Work out the finished part from the listing and answer in its coordinate system (mm). Coordinates: 2 decimals unless noted, no trailing zeros. Loops run counter-clockwise (first coordinate to the right, second up) from the corner with the lowest first, then second, coordinate; pieces in that order, holes last. Notation, with made-up numbers: (27, 45.5) - (78, 45.5) arc R21 ccw to (78, 79.5) - close; hole circle Ø10 at (70, -27). An arc over 180 degrees is marked (long way). Write each question's results on one line, items separated by ' | '. Start each with the question number.
1. A cutting plane is placed at B-B on x = -85. Determine the outline of the cut face in (y, z), then the cut area to 3 significant figures.
2. Each of these flat-tipped pins is pushed along its axis until it touches: P1, Ø10, axis at x = -74.5, y = 95, coming from the -Z side; P2, Ø1.6, axis at x = -62.7, y = 109.08, coming from the -Z side; P3, Ø2.5, axis at x = -121.2, y = 144.58, coming from the -Z side. Where does it stop, or does it pass through?
3. Find the intervals of material crossed by line 1 along Y through (x, z) = (-60, 0.3); line 2 along X through (y, z) = (54, 1); line 3 along Y through (x, z) = (-23.5, 0.6), in increasing order. Write a range as [from, to].
4. A cutting plane is placed at C-C on y = 39.5. Determine the outline of the cut face in (x, z).
5. A cutting plane is placed at A-A on z = 0.55. Determine the outline of the cut face in (x, y), then the cut area to 3 significant figures.
from build123d import *

# Parameters (mm, degrees)
SKETCH1_R           = 1
BOSS_EXTRUDE1_DEPTH = 1.5
CHAMFER1_SIZE       = 1


with BuildPart() as part:
    # Sketch1 → Boss-Extrude1 (new body)
    with BuildSketch(Plane.XY):
        with BuildLine():
            Line((20.7161288, 151.924941972), (-143.43387189, 151.924941972))
            ThreePointArc((-143.43387189, 151.924941972), (-144.494532062, 151.485602143), (-144.93387189, 150.424941972))
            Line((-144.93387189, 150.424941972), (-144.93387189, 48.261817052))
            ThreePointArc((-144.93387189, 48.261817052), (-144.494532062, 47.20115688), (-143.43387189, 46.761817052))
            Line((-143.43387189, 46.761817052), (-38.493629317, 46.761817052))
            ThreePointArc((-38.493629317, 46.761817052), (-37.328943614, 46.60848327), (-36.243629317, 46.158931369))
            Line((-36.243629317, 46.158931369), (-4.017847382, 27.553367493))
            ThreePointArc((-4.017847382, 27.553367493), (-2.879618836, 27.403516854), (-1.968809299, 28.10240556))
            Line((-1.968809299, 28.10240556), (22.015166883, 69.64386796))
            ThreePointArc((22.015166883, 69.64386796), (22.165017534, 70.005639409), (22.2161288, 70.393867999))
            Line((22.2161288, 70.393867999), (22.2161288, 150.424941972))
            ThreePointArc((22.2161288, 150.424941972), (21.776788972, 151.485602143), (20.7161288, 151.924941972))
        make_face()
        with Locations((-24.69657117, 144.575050352)):
            Circle(SKETCH1_R, mode=Mode.SUBTRACT)
        with Locations((-121.19657121, 144.575050352)):
            Circle(SKETCH1_R, mode=Mode.SUBTRACT)
        with Locations((-62.69657137, 109.075050232)):
            Circle(SKETCH1_R, mode=Mode.SUBTRACT)
        with Locations((-102.19657111, 52.825050972)):
            Circle(SKETCH1_R, mode=Mode.SUBTRACT)
        with Locations((-1.69657145, 53.825048972)):
            Circle(SKETCH1_R, mode=Mode.SUBTRACT)
    extrude(amount=BOSS_EXTRUDE1_DEPTH)

    # Chamfer1
    chamfer1_edges = [part.edges().sort_by_distance(p)[0] for p in [
        (-25.69657117, 144.575050352, 0),
        (-122.19657121, 144.575050352, 0),
        (-63.69657137, 109.075050232, 0),
        (-103.19657111, 52.825050972, 0),
        (-2.69657145, 53.825048972, 0),
    ]]
    chamfer(chamfer1_edges, length=CHAMFER1_SIZE)


solid = part.part
Values:
1) outline: (46.76, 0) - (151.92, 0) - (151.92, 1.5) - (46.76, 1.5) - close | area: 158 mm^2
2) P1: z = 0 | P2: through | P3: z = 0.74
3) line 1: [46.76, 151.92] | line 2: [-144.93, -2.68], [-0.71, 12.98] | line 3: [38.8, 143.85], [145.3, 151.92]
4) outline: (-24.71, 0) - (4.61, 0) - (4.61, 1.5) - (-24.71, 1.5) - close
5) outline: (-144.93, 48.26) arc R1.5 ccw to (-143.43, 46.76) - (-38.49, 46.76) arc R4.5 cw to (-36.24, 46.16) - (-4.02, 27.55) arc R1.5 ccw to (-1.97, 28.1) - (22.02, 69.64) arc R1.5 ccw to (22.22, 70.39) - (22.22, 150.42) arc R1.5 ccw to (20.72, 151.92) - (-143.43, 151.92) arc R1.5 ccw to (-144.93, 150.42) - close; hole circle Ø2.9 at (-121.2, 144.58); hole circle Ø2.9 at (-102.2, 52.83); hole circle Ø2.9 at (-62.7, 109.08); hole circle Ø2.9 at (-24.7, 144.58); hole circle Ø2.9 at (-1.7, 53.83) | area: 17,800 mm^2
